from build123d import *

# Parameters (mm, degrees)
BOSS_EXTRUDE2_DEPTH = 2
SKETCH2_R           = 2.425
CUT_EXTRUDE1_DEPTH  = 2


with BuildPart() as part:
    # Sketch1 → Boss-Extrude2 (new body)
    with BuildSketch(Plane.XY):
        with BuildLine():
            Line((2, 0), (22.85, 0))
            ThreePointArc((22.85, 0), (24.264213562, 0.585786438), (24.85, 2))
            Line((24.85, 2), (24.85, 30.85))
            ThreePointArc((24.85, 30.85), (24.264213562, 32.264213562), (22.85, 32.85))
            Line((22.85, 32.85), (2, 32.85))
            ThreePointArc((2, 32.85), (0.585786438, 32.264213562), (0, 30.85))
            Line((0, 30.85), (0, 2))
            ThreePointArc((0, 2), (0.585786438, 0.585786438), (2, 0))
        make_face()
    extrude(amount=BOSS_EXTRUDE2_DEPTH)

    # Sketch2 → Cut-Extrude1 (cut)
    with BuildSketch(Plane.XY.offset(2)):
        with Locations((4.425, 4.425)):
            Circle(SKETCH2_R)
        with Locations((12.425, 4.425)):
            Circle(SKETCH2_R)
        with Locations((20.425, 4.425)):
            Circle(SKETCH2_R)
        with Locations((4.425, 12.425)):
            Circle(SKETCH2_R)
        with Locations((12.425, 12.425)):
            Circle(SKETCH2_R)
        with Locations((20.425, 12.425)):
            Circle(SKETCH2_R)
        with Locations((4.425, 20.425)):
            Circle(SKETCH2_R)
        with Locations((12.425, 20.425)):
            Circle(SKETCH2_R)
        with Locations((20.425, 20.425)):
            Circle(SKETCH2_R)
        with Locations((4.425, 28.425)):
            Circle(SKETCH2_R)
        with Locations((12.425, 28.425)):
            Circle(SKETCH2_R)
        with Locations((20.425, 28.425)):
            Circle(SKETCH2_R)
    extrude(amount=-CUT_EXTRUDE1_DEPTH, mode=Mode.SUBTRACT)


solid = part.part
Work out the finished part from the listing and answer in its coordinate system (mm). Round coordinates to 2 decimals unless told otherwise and drop trailing zeros. Write each loop counter-clockwise with the first axis right and the second up, starting at its lowest first coordinate (ties: lowest second). Pieces come first, ordered by that corner, then holes.
1) A cutting plane is placed at B-B (y = 11). Give the vertices of the cut face in (x, z).
2) A cutting plane is placed at C-C (z = 1.55). Give the number of separate pieces and of enclosed holes in the cut face, plus the area to 3 significant figures.
3) A cutting plane is placed at A-A (x = 22). Give the vertices of the cut face in (y, z), plus the area to 3 significant figures.
4) Straight lines are drawn through the part: line 1 (X direction, y = 30.5, z = 1.6); line 2 (X direction, y = 28.5, z = 1.3); line 3 (Y direction, x = 12.75, z = 1.95). For each, find the intervals that lie inside material, in ascending order.
5) A cutting plane is placed at D-D (x = 11.75). Give the vertices of the cut face in (y, z).
6) The mould has two halves that part along Y. Classify faces 1 (the cylindrical face through (18.5, 10.95, 1.01)), 2 (the cylindrical face through (0.57, 0.6, 0.99)), 3 (the flat face through (24.85, 16, 1)): pulls with the +Y half, pulls with the -Y half, needs draft (parallel to the pull), parting line crosses it, or undercut.
Completed:
1. outline: (0, 0) - (2.46, 0) - (2.46, 2) - (0, 2) - close; (6.39, 0) - (10.46, 0) - (10.46, 2) - (6.39, 2) - close; (14.39, 0) - (18.46, 0) - (18.46, 2) - (14.39, 2) - close; (22.39, 0) - (24.85, 0) - (24.85, 2) - (22.39, 2) - close
2. separate pieces: 1
2. enclosed holes: 12
2. area: 591 mm2
3. outline: (0, 0) - (2.58, 0) - (2.58, 2) - (0, 2) - close; (6.27, 0) - (10.58, 0) - (10.58, 2) - (6.27, 2) - close; (14.27, 0) - (18.58, 0) - (18.58, 2) - (14.27, 2) - close; (22.27, 0) - (26.58, 0) - (26.58, 2) - (22.27, 2) - close; (30.27, 0) - (32.85, 0) - (32.85, 2) - (30.27, 2) - close
3. area: 36.2 mm2
4. line 1: x = 0 to 3.17, 5.68 to 11.17, 13.68 to 19.17, 21.68 to 24.85
4. line 2: x = 0 to 2, 6.85 to 10, 14.85 to 18, 22.85 to 24.85
4. line 3: y = 0 to 2.02, 6.83 to 10.02, 14.83 to 18.02, 22.83 to 26.02, 30.83 to 32.85
5. outline: (0, 0) - (2.1, 0) - (2.1, 2) - (0, 2) - close; (6.75, 0) - (10.1, 0) - (10.1, 2) - (6.75, 2) - close; (14.75, 0) - (18.1, 0) - (18.1, 2) - (14.75, 2) - close; (22.75, 0) - (26.1, 0) - (26.1, 2) - (22.75, 2) - close; (30.75, 0) - (32.85, 0) - (32.85, 2) - (30.75, 2) - close
6. face 1: undercut
6. face 2: pulls with the -Y half
6. face 3: needs draft
